from build123d import *

# Parameters (mm, degrees)
F0_W     = 20
F0_H     = 15
F1_DEPTH = 10
F3_R     = 2


# Not quite as in the source:
# - a feature of the source that left no trace in its solid (it failed there, or was rolled back) is left out


with BuildPart() as f1:
    # F0 (on Top) → F1 (new body)
    with BuildSketch(Plane.XY):
        Polygon((0, 24.5688632738), (-10, 6.7879746571), (10, 6.7879746571), align=None)
        with Locations((0, -0.7120253429)):
            Rectangle(F0_W, F0_H)
    extrude(amount=F1_DEPTH)

    # F3
    f3_edges = [f1.edges().sort_by_distance(p)[0] for p in [
        (-10, -0.712025, 0),
        (-5, 15.678419, 0),
        (0, 24.568863, 5),
        (-5, 15.678419, 10),
        (-10, -8.212025, 5),
        (-10, -0.712025, 10),
        (10, -8.212025, 5),
        (0, -8.212025, 0),
        (0, -8.212025, 10),
        (10, 6.787975, 5),
        (10, -0.712025, 0),
        (10, -0.712025, 10),
        (5, 15.678419, 0),
        (5, 15.678419, 10),
    ]]
    fillet(f3_edges, radius=F3_R)


solid = f1.part
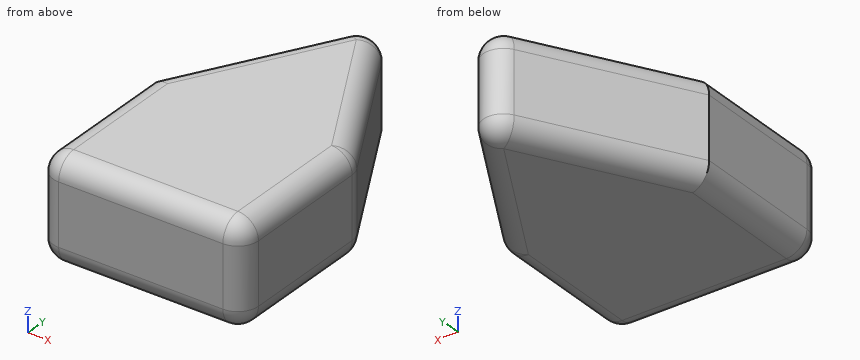
Can you work these out from the model? Positions are in its coordinate system, mm. Round coordinates to 2 decimals unless told otherwise and drop trailing zeros. Write each loop counter-clockwise with the first axis right and the second up, starting at its lowest first coordinate (ties: lowest second). Pieces come first, ordered by that corner, then holes. Notation, with made-up numbers: M 76,-28.5 L 117,-28.5 A8 ccw 117,-23.5 Z; hole C 44,7.25 d2. An arc over 180 degrees is marked long. Use CSV: the item, a comma, the result in double quotes.
(1) Imagine slicing it at B-B (z = 5.5). Write out the boundary of the cut face in (x, y).
Check values:
outline,"M -10,-6.21 A2 ccw -8,-8.21 L 8,-8.21 A2 ccw 10,-6.21 L 10,6.26 A2 ccw 9.74,7.24 L 1.74,21.47 A2 ccw -1.74,21.47 L -10,6.79 Z"
(2) Imagine slicing it at C-C (z = 1). Write out the boundary of the cut face in (x, y).
Check values:
outline,"M -9.73,-6.21 A1.73 ccw -8,-7.94 L 8,-7.94 A1.73 ccw 9.73,-6.21 L 9.73,6.26 A1.73 ccw 9.51,7.11 L 1.51,21.34 A1.73 ccw -1.51,21.34 L -9.73,6.72 Z"
(3) I'm going to push flat-ended pins straight in: pin 1 (6 mm diameter, centred on y = 7.5, z = 8.5, fed in from -X); pin 2 (1 mm diameter, centred on x = 4, z = 8.5, fed in from +Y); pin 3 (3 mm diameter, centred on x = -5, z = 1, fed in from +Y); pin 4 (3 mm diameter, centred on x = -6.5, z = 6, fed in from +Y). Where does each tip first touch, or does it pass through?
Check values:
pin 1,"x = -10"
pin 2,"y = 18.25"
pin 3,"y = 18.07"
pin 4,"y = 15.68"
(4) Imagine slicing it at A-A (y = 0.5). Write out the boundary of the cut face in (x, z).
Check values:
outline,"M -10,2 A2 ccw -8,0 L 8,0 A2 ccw 10,2 L 10,8 A2 ccw 8,10 L -8,10 A2 ccw -10,8 Z"
(5) I need wall thicknesses on line 1 along Y through (x, z) = (-2.5, 8.75); line 2 along X through (y, z) = (-3, 1); line 3 along Y through (x, z) = (0.25, 3.25). Which ranges of each line are inside material? Lowest first, please.
Check values:
line 1,"-8.07 to 19.83"
line 2,"-9.73 to 9.73"
line 3,"-8.21 to 22.47"
